Can you work these out from the model? Positions are in its coordinate system, mm. Give positions to 0.01 mm unless a question says otherwise; leave off trailing zeros. Order: outer loops, then holes, each group sorted by start corner. A loop starts at its lowest first (then second) coordinate and runs counter-clockwise, first axis right, second up. Notation, with made-up numbers: (46.5, 19) - (86.5, 19) arc R14 ccw to (86.5, 43) - close; hole circle Ø3 at (64, 16). An arc over 180 degrees is marked (long way). Answer as a JSON object with one key per item and string values.
```python
from build123d import *

# Parameters (mm, degrees)
SKETCH1_W           = 406.4
SKETCH1_H           = 279.4
BOSS_EXTRUDE1_DEPTH = 4.7625
SKETCH2_R           = 12.7
CUT_EXTRUDE1_DEPTH  = 4.7625
SKETCH3_R           = 2.032
CUT_EXTRUDE2_DEPTH  = 4.7625


with BuildPart() as part:
    # Sketch1 → Boss-Extrude1 (new body)
    with BuildSketch(Plane.XY):
        with Locations((-203.2, 139.7)):
            Rectangle(SKETCH1_W, SKETCH1_H)
    extrude(amount=BOSS_EXTRUDE1_DEPTH)

    # Sketch2 → Cut-Extrude1 (cut)
    with BuildSketch(Plane.XY.offset(4.7625)):
        with Locations((-203.2, 139.7)):
            Circle(SKETCH2_R)
    extrude(amount=-CUT_EXTRUDE1_DEPTH, mode=Mode.SUBTRACT)

    # Sketch3 → Cut-Extrude2 (cut)
    with BuildSketch(Plane(origin=(0, 0, 0), x_dir=(-1, 0, 0), z_dir=(0, 0, -1))):
        with Locations((203.2, 114.3)):
            Circle(SKETCH3_R)
        with Locations((203.2, 165.1)):
            Circle(SKETCH3_R)
    extrude(amount=-CUT_EXTRUDE2_DEPTH, mode=Mode.SUBTRACT)


solid = part.part
```
Q1. If we section it at A-A, the plane y = 139.7: Please give me the cut outline in (x, z).
Recorded:
{"outline": "(-406.4, 0) - (-215.9, 0) - (-215.9, 4.76) - (-406.4, 4.76) - close; (-190.5, 0) - (0, 0) - (0, 4.76) - (-190.5, 4.76) - close"}
Q2. We'd pull the mould along Y, two halves only. Please class faces 1 (the face through (-212.56, 148.283, 2.415)), 2 (the face through (-206, 111, 0)): released by +Y, released by -Y, zero draft, split by the parting line, or undercut.
Recorded:
{"face 1": "undercut", "face 2": "zero draft"}
Q3. I need wall thicknesses on L1, parallel to Y at x = -203.2, z = 3.6; L2, parallel to X at y = 165.1, z = 1.75; L3, parallel to Y at x = -197, z = 3.65. Which ranges of each line are inside material? Lowest first, please.
Recorded:
{"L1": "y = 0 to 112.27, 116.33 to 127, 152.4 to 163.07, 167.13 to 279.4", "L2": "x = -406.4 to -205.23, -201.17 to 0", "L3": "y = 0 to 128.62, 150.78 to 279.4"}
